The figure shows three views and two pictorial views of one solid part (mm, origin at its lowest corner). Answer the questions. A direction names the side the tool comes from. Round coordinates to 2 decimals unless told otherwise and drop trailing zeros. Order: outer loops, then holes, each group sorted by start corner. A loop starts at its lowest first (then second) coordinate and runs counter-clockwise, first axis right, second up. Notation, with made-up numbers: (4, -19) -> (27, -19) arc R10 ccw to (27, -7) -> close; hole circle Ø1 at (16.5, 40.5). An arc over 180 degrees is marked (long way). Return JSON: item names as keys, results as strings. Group by question number.
(1) Each of these flat-tipped pins is pushed along its axis until it touches: pin 1 (4 mm diameter, centred on x = 65.5, z = 5, fed in from +Y); pin 2 (10 mm diameter, centred on x = 96, y = 30, fed in from +Z); pin 3 (2.5 mm diameter, centred on x = 47.5, z = 6, fed in from -Y). Where does it stop, or does it pass through?
(2) The part is cut by section D-D (z = 5.5). Determine the outline of the cut face in (x, y), plus the area to 3 significant figures.
(3) Determine the mould class of the marked faces 1, 2 and 3 for opening direction X: +X half, -X half, draft (parallel to the pull), parting line (faces both ways), or undercut.
(4) Which of the six approach directions +Z, -Z, +X, -X, +Y, -Y give full straight-line access (tool end or side, diameter ignored) to the marked faces 4 and 5?
(5) The part is cut by section A-A (z = 29). Determine the outline of the cut face in (x, y), plus the area to 3 significant figures.
(6) The part is cut by section C-C (y = 69.5). Determine the outline of the cut face in (x, z), plus the area to 3 significant figures.
(7) Consider line 1 (X direction, y = 78.5, z = 28); line 2 (Y direction, x = 11, z = 25.5); line 3 (Z direction, x = 56, y = 74). Determine where each line is inside the solid, lowest interval first. Write a range as [from, to].
(8) The part is cut by section B-B (x = 44). Determine the outline of the cut face in (y, z).
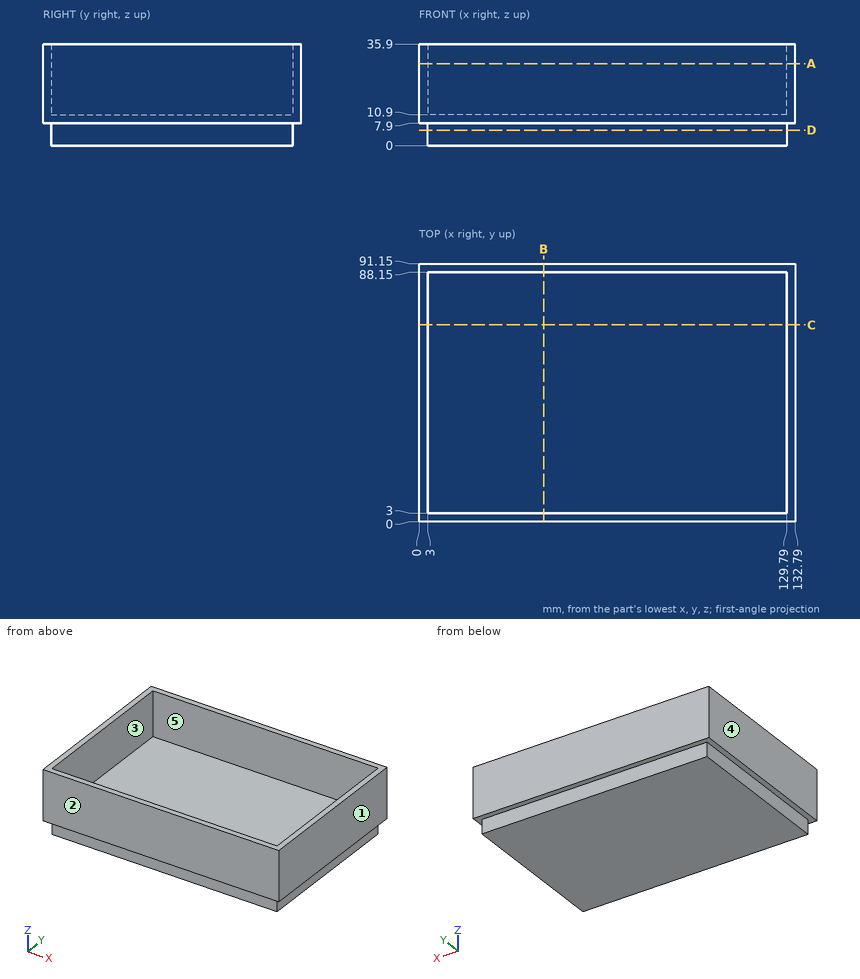
Answer below:
{
 "1": {"pin 1": "stops at y = 88.15", "pin 2": "stops at z = 10.9", "pin 3": "stops at y = 3"},
 "2": {"outline": "(3, 3) -> (129.79, 3) -> (129.79, 88.15) -> (3, 88.15) -> close", "area": "10,800 mm²"},
 "3": {"face 1": "+X half", "face 2": "draft", "face 3": "undercut"},
 "4": {"face 4": "+Z, -Z, -X, +Y, -Y", "face 5": "+Z"},
 "5": {"outline": "(0, 0) -> (132.79, 0) -> (132.79, 91.15) -> (0, 91.15) -> close; hole (3, 3) -> (129.79, 3) -> (129.79, 88.15) -> (3, 88.15) -> close", "area": "1,310 mm²"},
 "6": {"outline": "(0, 7.9) -> (3, 7.9) -> (3, 0) -> (129.79, 0) -> (129.79, 7.9) -> (132.79, 7.9) -> (132.79, 35.9) -> (129.79, 35.9) -> (129.79, 10.9) -> (3, 10.9) -> (3, 35.9) -> (0, 35.9) -> close", "area": "1,550 mm²"},
 "7": {"line 1": "x = [0, 3], [129.79, 132.79]", "line 2": "y = [0, 3], [88.15, 91.15]", "line 3": "z = [0, 10.9]"},
 "8": {"outline": "(0, 7.9) -> (3, 7.9) -> (3, 0) -> (88.15, 0) -> (88.15, 7.9) -> (91.15, 7.9) -> (91.15, 35.9) -> (88.15, 35.9) -> (88.15, 10.9) -> (3, 10.9) -> (3, 35.9) -> (0, 35.9) -> close"}
}
